```python
from build123d import *

# Parameters (mm, degrees)
SKETCH2_W           = 20.028
SKETCH2_H           = 20.028
SKETCH2_W_2         = 13.678
SKETCH2_H_2         = 13.678
BOSS_EXTRUDE2_DEPTH = 3.175
SKETCH2_3_W         = 25.4
SKETCH2_3_H         = 25.4
SKETCH2_3_W_2       = 20.028
SKETCH2_3_H_2       = 20.028
SKETCH2_3_W_3       = 13.678
SKETCH2_3_H_3       = 13.678
BOSS_EXTRUDE3_DEPTH = 3.175
FILLET1_R           = 2.54
CUT_EXTRUDE1_DEPTH  = 33.278974844


with BuildPart() as part:
    # Sketch2 → Boss-Extrude2 (new body)
    with BuildSketch(Plane(origin=(0, 0, 0), x_dir=(1, 0, 0), z_dir=(0, 1, 0))):
        with Locations((10.014, 10.014)):
            Rectangle(SKETCH2_W, SKETCH2_H)
        with Locations((10.014, 10.014)):
            Rectangle(SKETCH2_W_2, SKETCH2_H_2, mode=Mode.SUBTRACT)
    extrude(amount=-BOSS_EXTRUDE2_DEPTH)

    # Sketch2_3 → Boss-Extrude3 (add)
    # profile 1 of 3: a face of its own
    with BuildSketch(Plane(origin=(0, 0, 0), x_dir=(1, 0, 0), z_dir=(0, 1, 0))):
        with Locations((10.014, 10.014)):
            Rectangle(SKETCH2_3_W, SKETCH2_3_H)
        with Locations((10.014, 10.014)):
            Rectangle(SKETCH2_3_W_2, SKETCH2_3_H_2, mode=Mode.SUBTRACT)
    # profile 2 of 3: a face of its own
    with BuildSketch(Plane(origin=(0, 0, 0), x_dir=(1, 0, 0), z_dir=(0, 1, 0))):
        with Locations((10.014, 10.014)):
            Rectangle(SKETCH2_3_W_2, SKETCH2_3_H_2)
        with Locations((10.014, 10.014)):
            Rectangle(SKETCH2_3_W_3, SKETCH2_3_H_3, mode=Mode.SUBTRACT)
    # profile 3 of 3: a face of its own
    with BuildSketch(Plane(origin=(0, 0, 0), x_dir=(1, 0, 0), z_dir=(0, 1, 0))):
        with Locations((10.014, 10.014)):
            Rectangle(SKETCH2_3_W_3, SKETCH2_3_H_3)
    extrude(amount=BOSS_EXTRUDE3_DEPTH)

    # Fillet1
    fillet1_edges = [part.edges().sort_by_distance(p)[0] for p in [
        (22.714, 3.175, -10.014),
        (10.014, 3.175, -22.714),
        (-2.686, 3.175, -10.014),
        (10.014, 3.175, 2.686),
    ]]
    fillet(fillet1_edges, radius=FILLET1_R)

    # Sketch3 → Cut-Extrude1 (cut, through all)
    with BuildSketch(Plane.XY):
        Polygon((0, -0.4), (0.4, 0), (0, 0), align=None)
        Polygon((20.028, -0.4), (19.628, 0), (20.028, 0), align=None)
    extrude(amount=-CUT_EXTRUDE1_DEPTH, mode=Mode.SUBTRACT)


solid = part.part
```
Could you check a few things on this model? Use its own coordinates, in mm. A direction names the side the tool comes from. Give positions to 0.01 mm unless a question says otherwise; leave off trailing zeros. Loops run counter-clockwise (first coordinate to the right, second up) from the corner with the lowest first, then second, coordinate; pieces in that order, holes last. Notation, with made-up numbers: (6, 13) -> (28, 13) arc R10 cw to (28, 23) -> close; hole circle Ø6 at (60.25, 22.5). An arc over 180 degrees is marked (long way). Put each result on its own line as item: value.
(1) For faces 5 (the face through (10, -2, -20.028)), 6 (the face through (10, -2, 0)), 7 (the face through (0, -2, -10)), 8 (the face through (10, -2, -3.175)), 9 (the face through (20.028, -2, -10)), which set-ups out of +Z, -Z, +X, -X, +Y, -Y let a thin tool reach every point of the face, with its end or its side?
Computed:
face 5: -Z, +X, -X, -Y
face 6: +Z, +X, -X, -Y
face 7: +Z, -Z, -X, -Y
face 8: -Y
face 9: +Z, -Z, +X, -Y
(2) Thinking about a two-plate mould opening in Z: for faces 1 (the face through (10, 0, -10)), 2 (the face through (10.2, 2.4, -22)), 3 (the face through (3.175, -2, -10)), 4 (the face through (1, -3.175, -10)), which applies, pulls with the +Z half, pulls with the -Z half, needs draft (parallel to the pull), parting line crosses it, or undercut?
Computed:
face 1: undercut
face 2: pulls with the -Z half
face 3: undercut
face 4: needs draft
(3) Imagine slicing it at C-C on z = -11.5. Write out the boundary of the cut face in (x, y) (3 decimals), plus the area to 3 significant figures.
Computed:
outline: (-2.686, 0) -> (0.4, 0) -> (0, -0.4) -> (0, -3.175) -> (3.175, -3.175) -> (3.175, 0) -> (16.853, 0) -> (16.853, -3.175) -> (20.028, -3.175) -> (20.028, -0.4) -> (19.628, 0) -> (22.714, 0) -> (22.714, 0.635) arc R2.54 ccw to (20.174, 3.175) -> (-0.146, 3.175) arc R2.54 ccw to (-2.686, 0.635) -> close
area: 97.9 mm^2
(4) Imagine slicing it at B-B on x = 12.75. Write out the boundary of the cut face in (y, z) (3 decimals), plus the area to 3 significant figures.
Computed:
outline: (-3.175, -20.028) -> (0, -20.028) -> (0, -22.714) -> (0.635, -22.714) arc R2.54 ccw to (3.175, -20.174) -> (3.175, 0.146) arc R2.54 ccw to (0.635, 2.686) -> (0, 2.686) -> (0, 0) -> (-3.175, 0) -> (-3.175, -3.175) -> (0, -3.175) -> (0, -16.853) -> (-3.175, -16.853) -> close
area: 98.0 mm^2
(5) Imagine slicing it at D-D on x = 2.5. Write out the boundary of the cut face in (y, z) (3 decimals), plus the area to 3 significant figures.
Computed:
outline: (-3.175, -20.028) -> (0, -20.028) -> (0, -22.714) -> (0.635, -22.714) arc R2.54 ccw to (3.175, -20.174) -> (3.175, 0.146) arc R2.54 ccw to (0.635, 2.686) -> (0, 2.686) -> (0, 0) -> (-3.175, 0) -> close
area: 141 mm^2
(6) Please list where these lines run through material, in increasing order: probe 1 along X at (y, z) = (-1, -7.5) (3 decimals); probe 2 along Y at (x, z) = (16.75, -4) (3 decimals); probe 3 along Z at (x, y) = (19, -2.5). Write a range as [from, to].
Computed:
probe 1: [0, 3.175], [16.853, 20.028]
probe 2: [0, 3.175]
probe 3: [-20.03, 0]
(7) Imagine slicing it at A-A on y = -2.5. Write out the boundary of the cut face in (x, z) (3 decimals).
Computed:
outline: (0, -20.028) -> (20.028, -20.028) -> (20.028, 0) -> (0, 0) -> close; hole (3.175, -16.853) -> (16.853, -16.853) -> (16.853, -3.175) -> (3.175, -3.175) -> close
(8) I'm going to push flat-ended pins straight in: pin 1 Ø3.5 at (x, y) = (9.5, -2) entering from -Z; pin 2 Ø1.6 at (x, y) = (8, -1.5) entering from +Z; pin 3 Ø2 at (y, z) = (-2.5, -7.5) entering from -X; pin 4 Ø15 at (x, z) = (9.5, -8) entering from -Y (3 decimals). Where does each tip first touch, or does it pass through?
Computed:
pin 1: z = -20.03
pin 2: z = 0
pin 3: x = 0
pin 4: y = -3.175
